Part print with two shaded views. Sizes in mm from the minimum x, y, z corner. Coordinates: 2 decimals unless noted, no trailing zeros. Write each loop counter-clockwise with the first axis right and the second up, starting at its lowest first coordinate (ties: lowest second). Pieces come first, ordered by that corner, then holes.
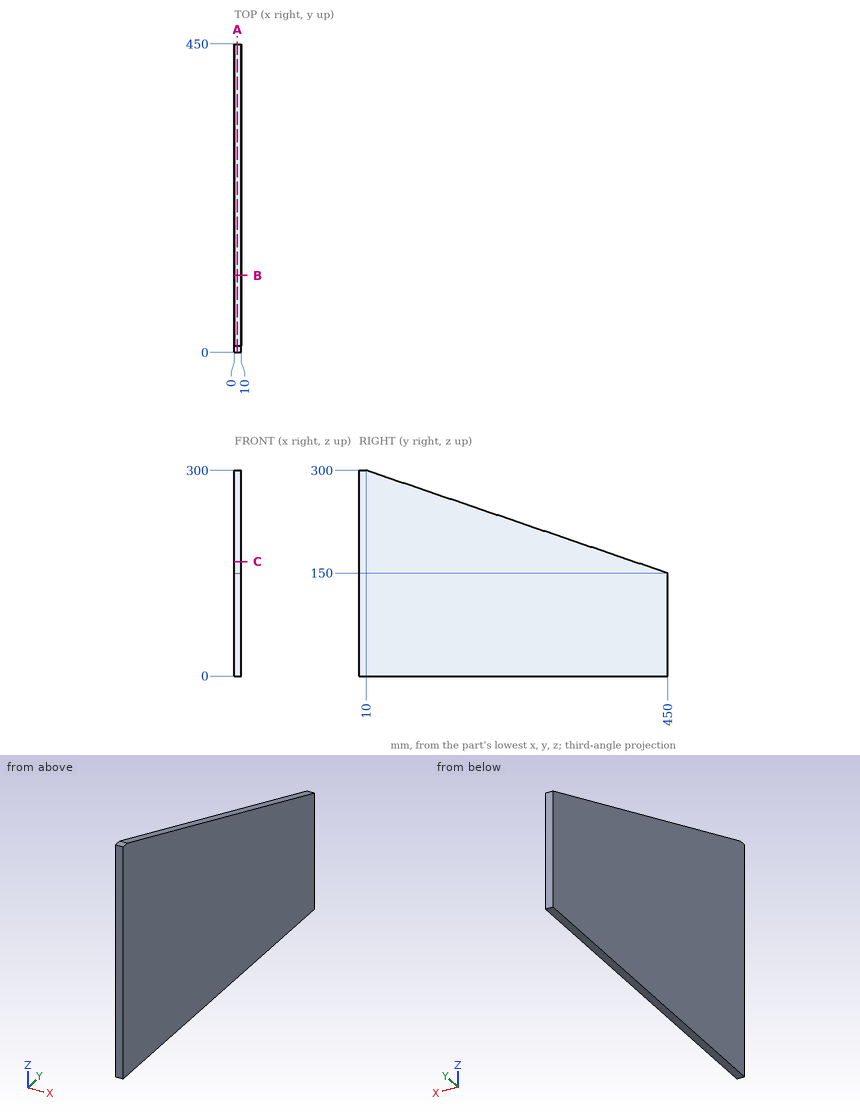
(1) Slice it at A-A, the plane x = 4.25. List the corners of the cut face in (y, z).
(2) Slice it at C-C, the plane z = 167. List the corners of the cut face in (x, y), and give its area (3 significant figures).
(3) Slice it at B-B, the plane y = 112.5. List the corners of the cut face in (x, z), and give its area (3 significant figures).
(4) Probe L1, parallel to Z at x = 1.25, y = 348.5; L2, parallel to Z at x = 9.75, y = 305. List the from-to ranges inside material, lowest first.
Results:
1. outline: (0, 0) - (450, 0) - (450, 150) - (10, 300) - (0, 300) - close
2. outline: (0, 0) - (10, 0) - (10, 400.13) - (0, 400.13) - close
2. area: 4,000 mm2
3. outline: (0, 0) - (10, 0) - (10, 265.06) - (0, 265.06) - close
3. area: 2,650 mm2
4. L1: z = 0 to 184.6
4. L2: z = 0 to 199.43
